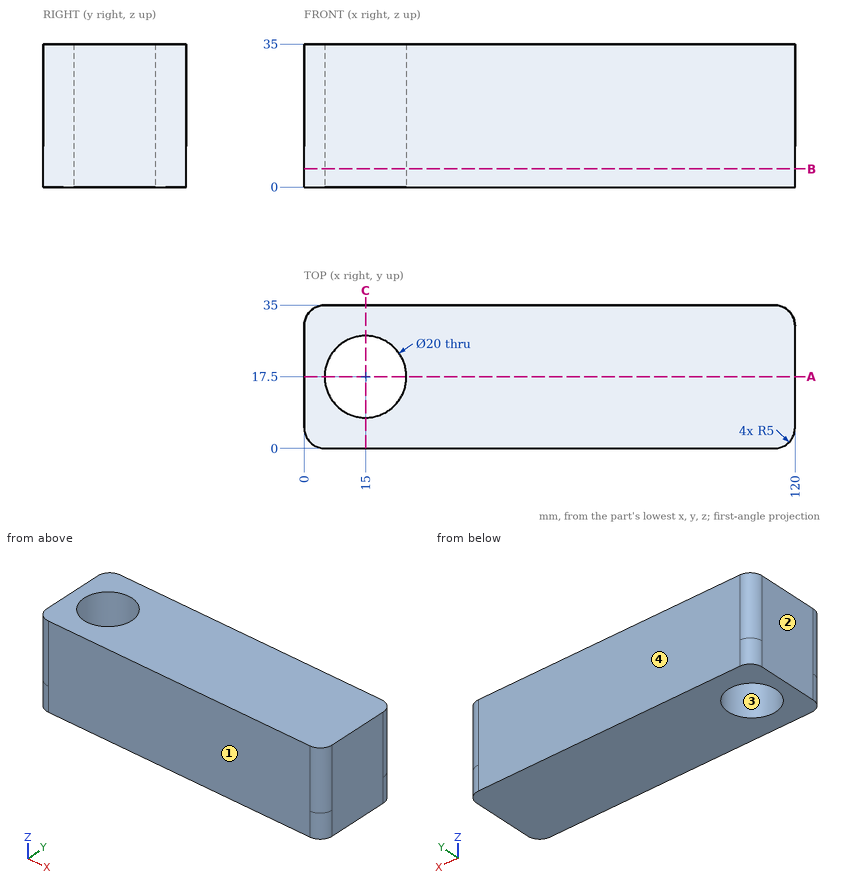
Job drawing, mm, ordinate dimensions from the low corner. One solid piece. Round coordinates to 2 decimals unless told otherwise and drop trailing zeros. Order: outer loops, then holes, each group sorted by start corner. A loop starts at its lowest first (then second) coordinate and runs counter-clockwise, first axis right, second up. Notation, with made-up numbers: (27.5, -5.75) -> (63.5, -5.75) arc R24 cw to (63.5, 6.25) -> close; hole circle Ø3 at (83.5, -20). An arc over 180 degrees is marked (long way). Answer in a Markdown table with one row per item.
1) Mould opens along Y. For the marked faces 1, 2, 3 and 4 say: released by +Y, released by -Y, zero draft, split by the parting line, or undercut.
Values:
| item | result |
|---|---|
| face 1 | released by -Y |
| face 2 | zero draft |
| face 3 | undercut |
| face 4 | released by +Y |
2) Band-saw the part on A-A on y = 17.5. Give the cut face in (x, z).
Values:
| item | result |
|---|---|
| outline | (0, 0) -> (5, 0) -> (5, 35) -> (0, 35) -> close; (25, 0) -> (120, 0) -> (120, 35) -> (25, 35) -> close |
3) Band-saw the part on C-C on x = 15. Give the cut face in (y, z), and give its area (3 significant figures).
Values:
| item | result |
|---|---|
| outline | (0, 0) -> (7.5, 0) -> (7.5, 35) -> (0, 35) -> close; (27.5, 0) -> (35, 0) -> (35, 35) -> (27.5, 35) -> close |
| area | 525 mm2 |
4) Wall check: L1, parallel to Y at x = 15, z = 14; L2, parallel to X at y = 17, z = 21; L3, parallel to Y at x = 115.5, z = 3.5. Give the ranges that are in metal, low to high.
Values:
| item | result |
|---|---|
| L1 | 0 to 7.5, 27.5 to 35 |
| L2 | 0 to 5.01, 24.99 to 120 |
| L3 | 0.03 to 34.97 |
5) Band-saw the part on B-B on z = 4.5. Give the cut face in (x, y).
Values:
| item | result |
|---|---|
| outline | (0, 5) arc R5 ccw to (5, 0) -> (115, 0) arc R5 ccw to (120, 5) -> (120, 30) arc R5 ccw to (115, 35) -> (5, 35) arc R5 ccw to (0, 30) -> close; hole circle Ø20 at (15, 17.5) |
